from build123d import *

# Parameters (mm, degrees)
SKETCH1_W               = 38.1
SKETCH1_H               = 16.764
BOSS_EXTRUDE1_DEPTH     = 25.4
CUT_EXTRUDE1_DEPTH      = 33.837789572
CUT_EXTRUDE3_DEPTH      = 33.837789572
CUT_EXTRUDE4_DEPTH      = 17.145
SKETCH7_R               = 2.159
CUT_EXTRUDE5_DEPTH      = 36.903957943
CUT_EXTRUDE6_DEPTH      = 34.822319923
CUT_EXTRUDE6_DEPTH_BACK = 34.822319923
SKETCH10_R              = 1.5875
CUT_EXTRUDE7_DEPTH      = 9.398


with BuildPart() as part:
    # Sketch1 → Boss-Extrude1 (new body)
    with BuildSketch(Plane(origin=(0, 0, 0), x_dir=(1, 0, 0), z_dir=(0, 1, 0))):
        Rectangle(SKETCH1_W, SKETCH1_H)
    extrude(amount=BOSS_EXTRUDE1_DEPTH)

    # Sketch3 → Cut-Extrude1 (cut, through all)
    with BuildSketch(Plane.XZ):
        Polygon((-2.54, 8.382), (-19.05, -5.132614164), (-19.05, 8.382), align=None)
        Polygon((19.05, -5.132614164), (19.05, 8.382), (2.54, 8.382), align=None)
    extrude(amount=-CUT_EXTRUDE1_DEPTH, mode=Mode.SUBTRACT)

    # Sketch5 → Cut-Extrude3 (cut, through all)
    with BuildSketch(Plane.XZ):
        with BuildLine():
            Line((-4.191, -5.132614164), (-15.113, -5.132614164))
            Line((-15.113, -5.132614164), (-5.790995153, 2.428103634))
            ThreePointArc((-5.790995153, 2.428103634), (-3.098385632, 2.748373809), (-1.651, 0.455385836))
            Line((-1.651, 0.455385836), (-1.651, -2.592614164))
            ThreePointArc((-1.651, -2.592614164), (-2.394948776, -4.388665388), (-4.191, -5.132614164))
        make_face()
        with BuildLine():
            Line((1.651, 0.455385836), (1.651, -2.592614164))
            ThreePointArc((1.651, -2.592614164), (2.394948776, -4.388665388), (4.191, -5.132614164))
            Line((4.191, -5.132614164), (15.113, -5.132614164))
            Line((15.113, -5.132614164), (5.790995153, 2.428103634))
            ThreePointArc((5.790995153, 2.428103634), (3.098385632, 2.748373809), (1.651, 0.455385836))
        make_face()
    extrude(amount=-CUT_EXTRUDE3_DEPTH, mode=Mode.SUBTRACT)

    # Sketch6 → Cut-Extrude4 (cut)
    with BuildSketch(Plane(origin=(0, 25.4, 0), x_dir=(1, 0, 0), z_dir=(0, 1, 0))):
        Polygon((1.651, -0.455385836), (1.651, -11.682968512), (19.05, 5.132614164), (4.191, 5.132614164), align=None)
        Polygon((-4.191, 5.132614164), (-1.651, -0.455385836), (-1.651, -11.682968512), (-19.05, 5.132614164), align=None)
    extrude(amount=-CUT_EXTRUDE4_DEPTH, mode=Mode.SUBTRACT)

    # Sketch7 → Cut-Extrude5 (cut, through all)
    with BuildSketch(Plane(origin=(0, 0, -8.382), x_dir=(-1, 0, 0), z_dir=(0, 0, -1))):
        with Locations((-9.398, 12.7)):
            Circle(SKETCH7_R)
        with Locations((9.398, 12.7)):
            Circle(SKETCH7_R)
    extrude(amount=-CUT_EXTRUDE5_DEPTH, mode=Mode.SUBTRACT)

    # Sketch9 → Cut-Extrude6 (cut, two sides: drawn at the far end of the back side and taken through both)
    with BuildSketch(Plane(origin=(1.651, 0, 0), x_dir=(0, 0, -1), z_dir=(1, 0, 0)).offset(-CUT_EXTRUDE6_DEPTH_BACK)):
        Polygon((5.132614164, 25.4), (-7.56675082, 8.255), (-10.075287768, 8.255), (-10.075287768, 25.4), (-7.56675082, 25.4), align=None)
    extrude(amount=CUT_EXTRUDE6_DEPTH + CUT_EXTRUDE6_DEPTH_BACK, mode=Mode.SUBTRACT)

    # Sketch10 → Cut-Extrude7 (cut)
    with BuildSketch(Plane.XY.offset(8.382)):
        with Locations((0, 4.623103893)):
            Circle(SKETCH10_R)
    extrude(amount=-CUT_EXTRUDE7_DEPTH, mode=Mode.SUBTRACT)


solid = part.part
Can you work these out from the model? Positions are in its coordinate system, mm. A direction names the side the tool comes from. Give positions to 0.01 mm unless a question says otherwise; leave off trailing zeros. Loops run counter-clockwise (first coordinate to the right, second up) from the corner with the lowest first, then second, coordinate; pieces in that order, holes last. Notation, with made-up numbers: (84, -35.5) -> (130, -35.5) arc R34 ccw to (130, -2.5) -> close; hole circle Ø3 at (-28, -22.5). An arc over 180 degrees is marked (long way). Return JSON: item names as keys, results as strings.
Q1. I need wall thicknesses on probe 1 along Z at (x, y) = (8.5, 17.25); probe 2 along Y at (x, z) = (2, 3.25) (3 decimals); probe 3 along X at (y, z) = (9.5, 4.5). Which ranges of each line are inside material? Lowest first, please.
Checks:
{"probe 1": "z = -8.38 to -5.13", "probe 2": "y = 0 to 8.255", "probe 3": "x = -1.65 to 1.65"}
Q2. I want a section at D-D, the plane z = -7.25. List the corners of the cut face in (x, y) for me.
Checks:
{"outline": "(-19.05, 0) -> (19.05, 0) -> (19.05, 25.4) -> (-19.05, 25.4) -> close; hole circle Ø4.32 at (-9.4, 12.7); hole circle Ø4.32 at (9.4, 12.7)"}
Q3. I want a section at A-A, the plane z = -0.5. List the corners of the cut face in (x, y) for me (1 decimal).
Checks:
{"outline": "(-13.4, 0) -> (-9.4, 0) -> (-9.4, 8.3) -> (-13.4, 8.3) -> close; (-1.7, 0) -> (1.7, 0) -> (1.7, 19.1) -> (-1.7, 19.1) -> close; (9.4, 0) -> (13.4, 0) -> (13.4, 8.3) -> (9.4, 8.3) -> close; hole circle Ø3.2 at (0, 4.6)"}
Q4. For pin 1 Ø10 at (x, y) = (-5.5, 5.5) entering from +Z; pin 2 Ø3 at (y, z) = (14.5, 2) entering from -X; pin 3 Ø8 at (x, y) = (9, 15) entering from +Z; pin 4 Ø2.5 at (x, y) = (0, 4.62) entering from +Z, each with a flat end and sliding along its axis, tell me the tip position at first contact or that it passes through.
Checks:
{"pin 1": "stops at z = 8.38", "pin 2": "stops at x = -1.65", "pin 3": "stops at z = -5.13", "pin 4": "stops at z = -1.02"}
Q5. I want a section at B-B, the plane x = 11. List the corners of the cut face in (y, z) for me (3 decimals), then the cut area to 4 significant figures.
Checks:
{"outline": "(0, -8.382) -> (11.253, -8.382) -> (11.253, -5.133) -> (0, -5.133) -> close; (0, -1.797) -> (8.255, -1.797) -> (8.255, 1.457) -> (0, 1.457) -> close; (14.147, -8.382) -> (25.4, -8.382) -> (25.4, -5.133) -> (14.147, -5.133) -> close", "area": "100.0 mm2"}
Q6. I want a section at C-C, the plane y = 12.7. List the corners of the cut face in (x, z) for me, then the cut area to 3 significant figures.
Checks:
{"outline": "(-19.05, -8.38) -> (-11.56, -8.38) -> (-11.56, -5.13) -> (-19.05, -5.13) -> close; (-7.24, -8.38) -> (7.24, -8.38) -> (7.24, -5.13) -> (4.19, -5.13) arc R2.54 cw to (1.65, -2.59) -> (1.65, 4.27) -> (-1.65, 4.27) -> (-1.65, -2.59) arc R2.54 cw to (-4.19, -5.13) -> (-7.24, -5.13) -> close; (11.56, -8.38) -> (19.05, -8.38) -> (19.05, -5.13) -> (11.56, -5.13) -> close", "area": "130 mm2"}
Q7. We'd pull the mould along Y, two halves only. Please class faces 4 (the face through (-3, 8.255, 3)), 5 (the face through (0, 5, -1.016)), 6 (the face through (-2.375, 12.522, -4.369)), 7 (the face through (9.9, 10.6, -6.8)): released by +Y, released by -Y, zero draft, split by the parting line, or undercut.
Checks:
{"face 4": "released by +Y", "face 5": "undercut", "face 6": "zero draft", "face 7": "undercut"}
Q8. On a 3-axis mill with a long thin cutter (end or side, diameter ignored), from which of +Z, -Z, +X, -X, +Y, -Y can I reach the whole of each face in a straight line? I mean faces 1 (the face through (1.651, 11, 0)), 2 (the face through (-19.05, 13, -7)), 3 (the face through (3.135, 4.07, 2.765)). Say none if no direction works.
Checks:
{"face 1": "+Y", "face 2": "+Z, -Z, -X, +Y, -Y", "face 3": "+Y, -Y"}
